Source: CAD feature listing. Evaluate the final solid. Frame: model axes, mm. A direction names the side the tool comes from. Give positions to 0.01 mm unless a question says otherwise; leave off trailing zeros. Loops run counter-clockwise (first coordinate to the right, second up) from the corner with the lowest first, then second, coordinate; pieces in that order, holes last. Notation, with made-up numbers: (64.25, 71) - (94.25, 71) arc R33 ccw to (94.25, 104) - close; hole circle Ø5 at (9, 71.25). An arc over 180 degrees is marked (long way). Put each result on its own line as item: value.
```python
from build123d import *


with BuildPart() as f2:
    # F2: sweep along a path in F1
    with BuildLine(Plane.XY) as f2_path:
        Line((111.1026118188, -65.109723053), (55.505612987, -31.187103672))
        Line((55.505612987, -31.187103672), (57.0849637179, 33.922619381))
        Line((57.0849637179, 33.922619381), (114.2613132806, 65.109723053))
        Line((114.2613132806, 65.109723053), (169.8583121124, 31.187103672))
        Line((169.8583121124, 31.187103672), (168.2789613815, -33.922619381))
        Line((168.2789613815, -33.922619381), (111.1026118188, -65.109723053))
    # F0 (on Front) → F2 (sweep)
    with BuildSketch(Plane.XZ):
        Polygon((-12.6929697398, -52.8973966771), (17.9204861451, -51.3624593682), (42.8443142989, -33.5203041197), (54.1653753864, -5.0356891564), (48.2893125029, 25.0477215336), (27.0817340957, 47.1786576154), (-2.7241035365, 54.3307032528), (-31.6650575434, 44.2331344899), (-50.5525795149, 20.0918580627), (-53.3900146779, -10.428441337), (-39.2764974165, -37.6377842961), align=None)
    sweep(path=f2_path.line, transition=Transition.RIGHT)


solid = f2.part
```
1) Mould query, pull axis Y, two halves, no side actions, for faces 4 (the flat face through (181.598, 110.035, 49.286)), 5 (the flat face through (146.745, 54.484, -19.515)), 6 (the flat face through (187.543, -140.398, -23.775)). Classes: pulls with the +Y half, pulls with the -Y half, needs draft (parallel to the pull), parting line crosses it, or undercut.
Check result:
face 4: pulls with the +Y half
face 5: undercut
face 6: pulls with the -Y half
2) Section query C-C, the plane x = 126. Output: boundary loops of the cut face in (y, z), plus the area to 3 significant figures.
Check result:
outline: (-181.85, -10.43) - (-165.78, -37.64) - (-135.51, -52.9) - (-100.65, -51.36) - (-72.26, -33.52) - (-59.37, -5.04) - (-66.06, 25.05) - (-90.21, 47.18) - (-124.15, 54.33) - (-157.11, 44.23) - (-178.62, 20.09) - close; (60.4, -5.04) - (73.66, -33.52) - (102.85, -51.36) - (138.7, -52.9) - (169.83, -37.64) - (186.36, -10.43) - (183.04, 20.09) - (160.92, 44.23) - (127.03, 54.33) - (92.12, 47.18) - (67.28, 25.05) - close
area: 20,300 mm²
3) Section query A-A, the plane z = 13.5. Output: boundary loops of the cut face in (x, y).
Check result:
outline: (-53.36, -90.57) - (108.1, -189.08) - (274.14, -98.51) - (278.73, 90.57) - (117.27, 189.08) - (-48.78, 98.51) - close; hole (49.71, -34.35) - (110.94, -71.71) - (173.91, -37.36) - (175.65, 34.35) - (114.42, 71.71) - (51.45, 37.36) - close
4) Pin query (flat end, axial travel): P1, Ø2, axis at x = 13.5, z = -29, coming from the +Y side; P2, Ø10, axis at x = 6.5, y = -25.5, coming from the -Z side; P3, Ø6, axis at x = 203.5, z = 38, coming from the -Y side. Return the tip coordinate at first contact, or that it passes through.
Check result:
P1: y = 124.85
P2: z = -52.15
P3: y = -123.53
5) Access query for faces 1 (the flat face through (28.5, -135, -23.8)), 2 (the flat face through (77.65, 66.21, 36.037)), 3 (the flat face through (156.61, 69.95, -42.67)). Directions: +Z, -Z, +X, -X, +Y, -Y. A direction counts if a zero-diameter tool reaches every point of the face in a straight line with its end or side. Return the directions, or none.
Check result:
face 1: -Z, -X, -Y
face 2: +Z
face 3: -Z
6) Section query D-D, the plane y = 125. Output: boundary loops of the cut face in (x, z).
Check result:
outline: (-4.86, -10.43) - (24.6, -37.64) - (80.1, -52.9) - (115.71, -52.04) - (148.45, -52.9) - (199.48, -37.64) - (226.57, -10.43) - (221.12, 20.09) - (184.87, 44.23) - (129.32, 54.33) - (115.71, 52.63) - (100.91, 54.33) - (40.49, 44.23) - (1.06, 20.09) - close
7) Material intervals for line 1 along Y through (x, z) = (67.5, -9); line 2 along Y through (x, z) = (170.5, 41); line 3 along X through (y, z) = (-32, -9.5), sorted ascending. Write a range as [from, to].
Check result:
line 1: [-166.76, -42.81], [43.79, 164.32]
line 2: [-135.72, -59.2], [58.03, 136.73]
line 3: [-54.08, 51.61], [172.2, 277.89]
8) Section query B-B, the plane y = 9. Output: boundary loops of the cut face in (x, z).
Check result:
outline: (-53.17, -10.43) - (-39.06, -37.64) - (-12.47, -52.9) - (18.14, -51.36) - (43.06, -33.52) - (54.38, -5.04) - (48.51, 25.05) - (27.3, 47.18) - (-2.51, 54.33) - (-31.45, 44.23) - (-50.33, 20.09) - close; (171.42, -5.04) - (182.74, -33.52) - (207.66, -51.36) - (238.28, -52.9) - (264.86, -37.64) - (278.97, -10.43) - (276.13, 20.09) - (257.25, 44.23) - (228.31, 54.33) - (198.5, 47.18) - (177.29, 25.05) - close
